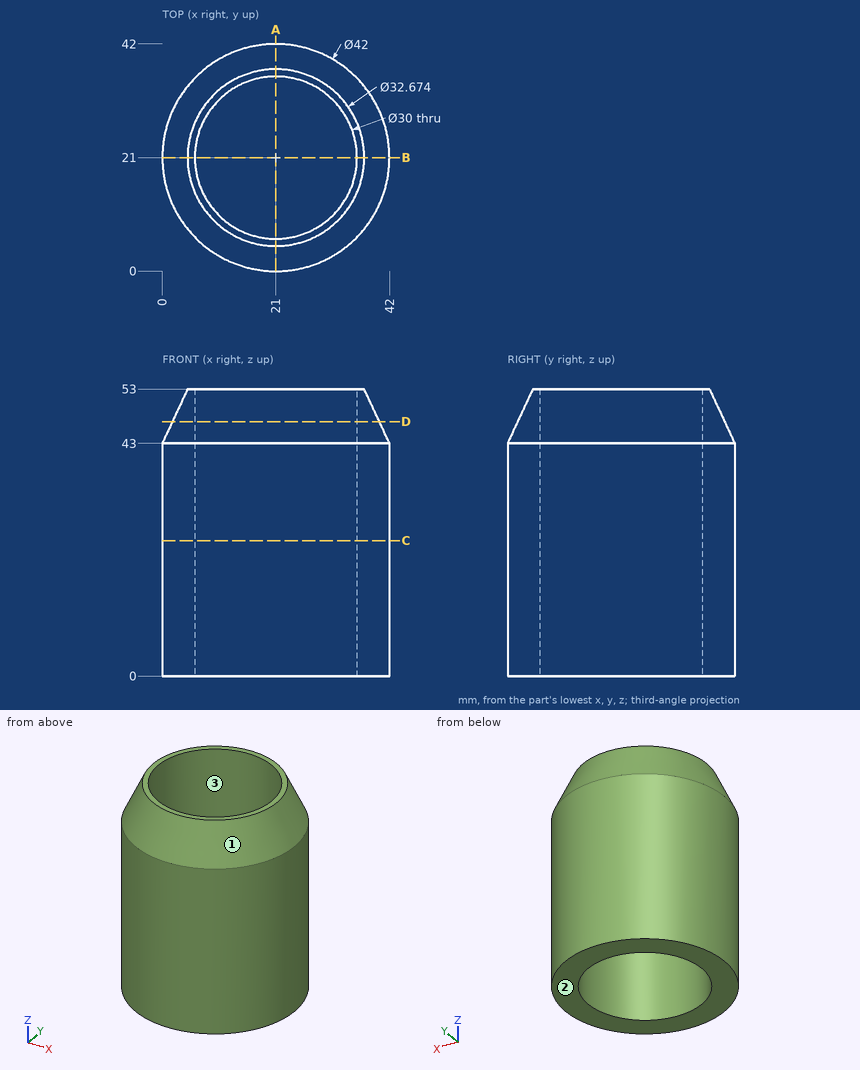
Geometry: see drawing. Coordinates: mm, zero at the bounding-box minimum. Give positions to 0.01 mm unless a question says otherwise; leave off trailing zeros. Loops run counter-clockwise (first coordinate to the right, second up) from the corner with the lowest first, then second, coordinate; pieces in that order, holes last. Notation, with made-up numbers: (28, 41) - (67, 41) arc R22 cw to (67, 64) - close; hole circle Ø1 at (72, 18). An arc over 180 degrees is marked (long way). Answer as CSV lines item,"result". Start each with the question number.
1. Section C-C, the plane z = 25. Return loops of the section in (x, y), plus the area to 3 significant figures.
2. Section A-A, the plane x = 21. Return loops of the section in (y, z), plus the area to 3 significant figures.
3. Pin query (flat end, axial travel): P1, Ø8, axis at x = 15, z = 15, coming from the +Y side; P2, Ø1, axis at y = 34, z = 40, coming from the -X side (1 decimal); P3, Ø18, axis at x = 21, y = 21, coming from the +Z side; P4, Ø4, axis at x = 5.5, z = 15.5, coming from the +Y side. Return the tip coordinate at first contact, or that it passes through.
4. Draft query along Y for the marked faces 1, 2 and 3. Return one class per face: released by +Y, released by -Y, zero draft, split by the parting line, or undercut.
5. Ray query, L1, parallel to Y at x = 21, z = 32; L2, parallel to Y at x = 32.5, z = 5; L3, parallel to X at y = 17, z = 9.5. Return the intervals inside material, ascending.
6. Section D-D, the plane z = 47. Return loops of the section in (x, y) (1 decimal).
Answers:
1,outline,"circle Ø42 at (21, 21); hole circle Ø30 at (21, 21)"
1,area,"679 mm2"
2,outline,"(0, 0) - (6, 0) - (6, 53) - (4.66, 53) - (0, 43) - close; (36, 0) - (42, 0) - (42, 43) - (37.34, 53) - (36, 53) - close"
2,area,"589 mm2"
3,P1,"stops at y = 41.9"
3,P2,"stops at x = 4.1"
3,P3,"passes through"
3,P4,"stops at y = 37.09"
4,face 1,"split by the parting line"
4,face 2,"zero draft"
4,face 3,"undercut"
5,L1,"y = 0 to 6, 36 to 42"
5,L2,"y = 3.43 to 11.37, 30.63 to 38.57"
5,L3,"x = 0.38 to 6.54, 35.46 to 41.62"
6,outline,"circle Ø38.3 at (21, 21); hole circle Ø30 at (21, 21)"
